Autodesk Inventor part; units mm, degrees
ref_plane "YZ Plane" through (0, 0, 0) normal (1, 0, 0) x (0, 1, 0)
ref_plane "XZ Plane" through (0, 0, 0) normal (0, 1, 0) x (-1, 0, 0)
ref_plane "XY Plane" through (0, 0, 0) normal (0, 0, 1) x (1, 0, 0)
sketch "Sketch5" plane through (0, 0, 0) normal (0, 1, 0) x (-1, 0, 0)
  line L0 (19.05, 9.525) -> (-19.05, 9.525)
  line L1 (-19.05, 9.525) -> (-19.05, -9.525)
  line L2 (-19.05, -9.525) -> (19.05, -9.525)
  line L3 (19.05, -9.525) -> (19.05, 9.525)
  line L4 (19.05, 9.525) -> (-19.05, -9.525) construction
  line L5 (-19.05, 9.525) -> (19.05, -9.525) construction
  line L6 (15.875, 6.35) -> (-15.875, 6.35)
  line L7 (-15.875, 6.35) -> (-15.875, -6.35)
  line L8 (-15.875, -6.35) -> (15.875, -6.35)
  line L9 (15.875, -6.35) -> (15.875, 6.35)
  line L10 (15.875, 6.35) -> (-15.875, -6.35) construction
  line L11 (-15.875, 6.35) -> (15.875, -6.35) construction
  point P0 (0, 0)
  dimension "d11" = 19.05
  dimension "d12" = 38.1
  dimension "d13" = 3.175
  dimension "d14" = 3.175
extrude "Extrusion4" add sketch "Sketch5" along normal blind 923.29
sketch "Sketch6" plane through (-19.05, 0, 9.525) normal (-1, 0, 0) x (0, 0, 1)
  circle A0 centre (-9.525, 821.69) radius 3.175
  line L0 (-19.05, 923.29) -> (0, 923.29)
  point P0 (-9.525, 0)
  dimension "d17" = 6.35
  dimension "d18" = 101.6
extrude "Extrusion6" cut sketch "Sketch6" against normal through all
equation "\"d11\" = tubeWidth"
equation "\"d12\" = tubeBreadth"
equation "\"d13\" = tubeMaterialThickness"
equation "\"d14\" = tubeMaterialThickness"
equation "\"d15\" = tubeLength"
equation "\"d17\" = endOfTravelPostDiam"
equation "\"d18\" = endOfTravellDistanceFromBottom"
equation "\"tubeBreadth\" = 38.1"
equation "\"tubeMaterialThickness\" = 3.175"
equation "\"tubeLength\" = 923.29"
equation "\"tubeWidth\" = 19.05"
equation "\"endOfTravelPostDiam\" = 6.35"
equation "\"endOfTravellDistanceFromBottom\" = 101.6"
properties part number "InnerTube" material "Aluminum 6061"
CAD build for the part. Positions are in the model's coordinates, mm. A direction names the side the tool comes from. Round coordinates to 2 decimals unless told otherwise and drop trailing zeros. Loops run counter-clockwise (first coordinate to the right, second up) from the corner with the lowest first, then second, coordinate; pieces in that order, holes last.
(1) Drop a flat-ended pin along its axis: pin 1 (4 mm diameter, centred on x = -13.5, z = -2, fed in from -Y) (1 decimal). Give the stop position or say it passes through.
(2) Wall check: line 1 along Z through (x, y) = (18.3, 821.69) (3 decimals); line 2 along Z through (x, y) = (-13, 686) (3 decimals); line 3 along X through (y, z) = (468, 0.75) (3 decimals). Give the ranges that are in metal, low to high.
(3) Cut at C-C (x = -2). Give the cut face in (y, z) (3 decimals), plus the area to 3 significant figures.
(4) Cut at B-B (y = 673). Give the cut face in (x, z) (3 decimals), plus the area to 3 significant figures.
(5) Cut at A-A (z = 0). Give the cut face in (x, y) (3 decimals), plus the area to 3 significant figures.
(6) Two-plate mould, pull along Z, no slides. Class faces 1 (the flat face through (0, 455, -6.35)), 2 (the flat face through (19.05, 455, 0)), 3 (the flat face through (0, 455, 9.525)): +Z half, -Z half, draft (parallel to the pull), parting line (faces both ways), or undercut.
(7) Which spindle directions (+Z, -Z, +X, -X, +Y, -Y) get a long thin tool onto all of the face, cutting with end or side? Do faces 4 (the flat face through (0, 455, 6.35)), 5 (the flat face through (0.3, 923.29, 6.5)). Say none if no direction does.
Findings below:
1. pin 1: passes through
2. line 1: z = -9.525 to -3.175, 3.175 to 9.525
2. line 2: z = -9.525 to -6.35, 6.35 to 9.525
2. line 3: x = -19.05 to -15.875, 15.875 to 19.05
3. outline: (0, -9.525) - (923.29, -9.525) - (923.29, -6.35) - (0, -6.35) - close; (0, 6.35) - (923.29, 6.35) - (923.29, 9.525) - (0, 9.525) - close
3. area: 5,860 mm2
4. outline: (-19.05, -9.525) - (19.05, -9.525) - (19.05, 9.525) - (-19.05, 9.525) - close; hole (-15.875, -6.35) - (15.875, -6.35) - (15.875, 6.35) - (-15.875, 6.35) - close
4. area: 323 mm2
5. outline: (-19.05, 0) - (-15.875, 0) - (-15.875, 818.515) - (-19.05, 818.515) - close; (-19.05, 824.865) - (-15.875, 824.865) - (-15.875, 923.29) - (-19.05, 923.29) - close; (15.875, 0) - (19.05, 0) - (19.05, 818.515) - (15.875, 818.515) - close; (15.875, 824.865) - (19.05, 824.865) - (19.05, 923.29) - (15.875, 923.29) - close
5. area: 5,820 mm2
6. face 1: undercut
6. face 2: draft
6. face 3: +Z half
7. face 4: +Y, -Y
7. face 5: +Z, -Z, +X, -X, +Y
